Here's how the part is built. I have some questions about the finished solid (model axes, mm). Face numbers are marked on the shaded views. Coordinates: 2 decimals unless noted, no trailing zeros. Write each loop counter-clockwise with the first axis right and the second up, starting at its lowest first coordinate (ties: lowest second). Pieces come first, ordered by that corner, then holes.
Item 1: Please list where these lines run through material, in increasing order: line 1 (Z direction, x = 0, y = 4.65); line 2 (X direction, y = 7.25, z = 4).
Item 2: I want a section at A-A (x = 0). Please give me the cut outline in (y, z).
Item 3: I want a section at B-B (z = 0). Please give me the cut outline in (x, y), and give its area (3 significant figures).
Item 4: If we mould it in two halves opening along X, with no side actions, what happens to the marked faces 1, 2 and 3? For each: pulls with the +X half, pulls with the -X half, needs draft (parallel to the pull), parting line crosses it, or undercut.
Item 5: I want a section at C-C (y = 10). Please give me the cut outline in (x, z), and give its area (3 significant figures).
Item 6: I'm going to push flat-ended pins straight in: P1, Ø6, axis at y = 7, z = 4, coming from the -X side; P2, Ø2, axis at x = -3.5, y = 7.5, coming from the -Z side. Where does each tip first touch, or does it pass through?
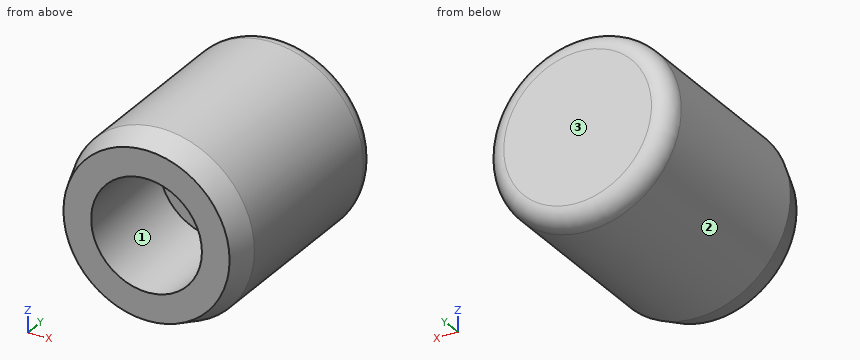
from build123d import *

# Parameters (mm, degrees)
SKETCH1_R           = 5
BOSS_EXTRUDE1_DEPTH = 12
SKETCH2_R           = 3
CUT_EXTRUDE1_DEPTH  = 6
FILLET1_R           = 1
CHAMFER1_SIZE       = 0.5
CHAMFER1_SIZE2      = 1.37373871


with BuildPart() as part:
    # Sketch1 → Boss-Extrude1 (new body)
    with BuildSketch(Plane(origin=(0, 0, 0), x_dir=(1, 0, 0), z_dir=(0, 1, 0))):
        Circle(SKETCH1_R)
    extrude(amount=BOSS_EXTRUDE1_DEPTH)

    # Sketch2 → Cut-Extrude1 (cut)
    with BuildSketch(Plane.XZ):
        Circle(SKETCH2_R)
    extrude(amount=-CUT_EXTRUDE1_DEPTH, mode=Mode.SUBTRACT)

    # Fillet1
    fillet1_edges = [part.edges().sort_by_distance(p)[0] for p in [
        (-5, 12, 0),
    ]]
    fillet(fillet1_edges, radius=FILLET1_R)

    # Chamfer1
    chamfer1_edges = [part.edges().sort_by_distance(p)[0] for p in [
        (-5, 0, 0),
    ]]
    chamfer1_side = [part.faces().sort_by_distance(p)[0] for p in [
        (-4.858578644, 0, 0),
    ]]
    chamfer(chamfer1_edges, length=CHAMFER1_SIZE, length2=CHAMFER1_SIZE2, reference=chamfer1_side[0])


solid = part.part
Answer:
1. line 1: z = -5 to -3, 3 to 5
1. line 2: x = -3 to 3
2. outline: (0, -4.5) - (1.37, -5) - (11, -5) arc R1 ccw to (12, -4) - (12, 4) arc R1 ccw to (11, 5) - (1.37, 5) - (0, 4.5) - (0, 3) - (6, 3) - (6, -3) - (0, -3) - close
3. outline: (-5, 1.37) - (-4.5, 0) - (-3, 0) - (-3, 6) - (3, 6) - (3, 0) - (4.5, 0) - (5, 1.37) - (5, 11) arc R1 ccw to (4, 12) - (-4, 12) arc R1 ccw to (-5, 11) - close
3. area: 82.9 mm2
4. face 1: undercut
4. face 2: parting line crosses it
4. face 3: needs draft
5. outline: circle Ø10 at (0, 0)
5. area: 78.5 mm2
6. P1: stops at x = -4.9
6. P2: stops at z = -4.33
